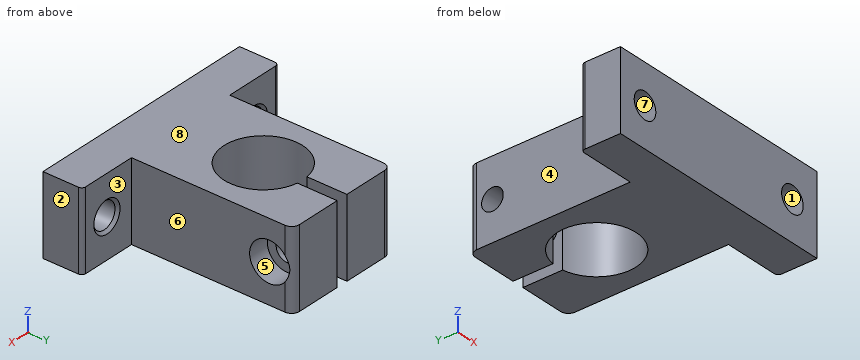
from build123d import *

# Parameters (mm, degrees)
BOSS_EXTRUDE1_DEPTH                                  = 20
CSK_FOR_M6_HEX_SOCKET_COUNTERSUNK_CAP_SC_D           = 6.6
CSK_FOR_M6_HEX_SOCKET_COUNTERSUNK_CAP_SC_CSINK_D     = 8
CSK_FOR_M6_HEX_SOCKET_COUNTERSUNK_CAP_SC_CSINK_ANGLE = 90
CBORE_FOR_M5_HEX_SOCKET_HEAD_CAP_SCREW1_D            = 5.5
CBORE_FOR_M5_HEX_SOCKET_HEAD_CAP_SCREW1_CBORE_D      = 10
CBORE_FOR_M5_HEX_SOCKET_HEAD_CAP_SCREW1_CBORE_DEPTH  = 5.4


with BuildPart() as part:
    # Sketch1 → Boss-Extrude1 (new body)
    with BuildSketch(Plane.XY):
        with BuildLine():
            Line((30, 0), (-30, 0))
            Line((-30, 0), (-30, 9))
            ThreePointArc((-30, 9), (-29.707106781, 9.707106781), (-29, 10))
            Line((-29, 10), (-15, 10))
            Line((-15, 10), (-15, 49))
            ThreePointArc((-15, 49), (-14.414213562, 50.414213562), (-13, 51))
            Line((-13, 51), (-1.5, 51))
            Line((-1.5, 51), (-1.5, 40.886859967))
            ThreePointArc((-1.5, 40.886859967), (0, 21), (1.5, 40.886859967))
            Line((1.5, 40.886859967), (1.5, 51))
            Line((1.5, 51), (13, 51))
            ThreePointArc((13, 51), (14.414213562, 50.414213562), (15, 49))
            Line((15, 49), (15, 10))
            Line((15, 10), (29, 10))
            ThreePointArc((29, 10), (29.707106781, 9.707106781), (30, 9))
            Line((30, 9), (30, 0))
        make_face()
    extrude(amount=BOSS_EXTRUDE1_DEPTH)

    # CSK for M6 Hex Socket Countersunk Cap Screw1 (through all)
    with Locations(Plane(origin=(-22.5, 10, 10), x_dir=(1, 0, 0), z_dir=(0, 1, 0))):
        with Locations((0, 0), (45, 0)):
            CounterSinkHole(CSK_FOR_M6_HEX_SOCKET_COUNTERSUNK_CAP_SC_D / 2, CSK_FOR_M6_HEX_SOCKET_COUNTERSUNK_CAP_SC_CSINK_D / 2, counter_sink_angle=CSK_FOR_M6_HEX_SOCKET_COUNTERSUNK_CAP_SC_CSINK_ANGLE)

    # CBORE for M5 Hex Socket Head Cap Screw1 (through all)
    with Locations(Plane(origin=(15, 45, 10), x_dir=(0, 0, 1), z_dir=(1, 0, 0))):
        with Locations((0, 0)):
            CounterBoreHole(CBORE_FOR_M5_HEX_SOCKET_HEAD_CAP_SCREW1_D / 2, CBORE_FOR_M5_HEX_SOCKET_HEAD_CAP_SCREW1_CBORE_D / 2, CBORE_FOR_M5_HEX_SOCKET_HEAD_CAP_SCREW1_CBORE_DEPTH)


solid = part.part
Verification items for the finished model (mm, model axes). Face numbers are marked on the shaded views. A direction names the side the tool comes from. Give positions to 0.01 mm unless a question says otherwise; leave off trailing zeros. Write each loop counter-clockwise with the first axis right and the second up, starting at its lowest first coordinate (ties: lowest second). Pieces come first, ordered by that corner, then holes.
(1) Cross-section at C-C (x = 22.5). Enter the section's corners in (y, z), plus the area to 3 significant figures.
(2) Gauge pin test, flat ends, axial feed: pin 1 (9 mm diameter, centred on y = 45, z = 10, fed in from +X); pin 2 (4 mm diameter, centred on x = 22, z = 6, fed in from +Y); pin 3 (6 mm diameter, centred on y = 35, z = 13.5, fed in from -X); pin 4 (5.5 mm diameter, centred on x = -22.5, z = 10, fed in from -Y). Record the tip position at first contact, or that the pin passes through.
(3) Mould release check, pull along X, two halves, no side actions. Record for the marked faces 6, 7 and 8: +X half, -X half, draft (parallel to the pull), parting line (faces both ways), or undercut.
(4) Material ranges on line 1 (X direction, y = 6, z = 10); line 2 (X direction, y = 41.5, z = 14.5); line 3 (Z direction, x = 3, y = 45), recorded low to high.
(5) Cross-section at D-D (y = 31). Enter the section's corners in (x, z), plus the area to 3 significant figures.
(6) Cross-section at A-A (x = -6). Enter the section's corners in (y, z).
(7) Cross-section at B-B (y = 45). Enter the section's corners in (x, z), plus the area to 3 significant figures.
(8) Access from +Z, -Z, +X, -X, +Y, -Y to the whole of each face (thin tool, end or side, straight path). Record for the marked faces 1, 2, 3, 4 and 5.
Worked out:
1. outline: (0, 0) - (10, 0) - (10, 6) - (9.3, 6.7) - (0, 6.7) - close; (0, 13.3) - (9.3, 13.3) - (10, 14) - (10, 20) - (0, 20) - close
1. area: 134 mm2
2. pin 1: stops at x = 9.6
2. pin 2: stops at y = 10
2. pin 3: stops at x = -15
2. pin 4: passes through
3. face 6: +X half
3. face 7: undercut
3. face 8: draft
4. line 1: x = -30 to -25.8, -19.2 to 19.2, 25.8 to 30
4. line 2: x = -15 to -1.5, 1.5 to 15
4. line 3: z = 0 to 7.25, 12.75 to 20
5. outline: (-15, 0) - (-10, 0) - (-10, 20) - (-15, 20) - close; (10, 0) - (15, 0) - (15, 20) - (10, 20) - close
5. area: 200 mm2
6. outline: (0, 0) - (23, 0) - (23, 20) - (0, 20) - close; (39, 0) - (51, 0) - (51, 20) - (39, 20) - close; hole circle Ø5.5 at (45, 10)
7. outline: (-15, 0) - (-1.5, 0) - (-1.5, 7.25) - (-15, 7.25) - close; (-15, 12.75) - (-1.5, 12.75) - (-1.5, 20) - (-15, 20) - close; (1.5, 0) - (15, 0) - (15, 5) - (9.6, 5) - (9.6, 7.25) - (1.5, 7.25) - close; (1.5, 12.75) - (9.6, 12.75) - (9.6, 15) - (15, 15) - (15, 20) - (1.5, 20) - close
7. area: 367 mm2
8. face 1: +Y, -Y
8. face 2: +Z, -Z, +X, +Y, -Y
8. face 3: +Z, -Z, +X, +Y
8. face 4: +Z, -Z, -X, +Y
8. face 5: +X
